Could you check a few things on this model? Use its own coordinates, in mm. Face numbers are marked on the shaded views. A direction names the side the tool comes from. Coordinates: 2 decimals unless noted, no trailing zeros. Write each loop counter-clockwise with the first axis right and the second up, starting at its lowest first coordinate (ties: lowest second). Pieces come first, ordered by that corner, then holes.
Item 1: I want a section at B-B on x = -133.5. Please give me the cut outline in (y, z).
Item 2: Thinking about a two-plate mould opening in Y: for the marked faces 1, 2 and 3, which applies, +Y half, -Y half, draft (parallel to the pull), parting line (faces both ways), or undercut?
Item 3: If I drill on probe 1 along Z at (x, y) = (35, 50); probe 2 along Y at (x, z) = (43.25, 45); probe 3 along X at (y, z) = (156, -101.5), over which ranges is the centre line in solid material (lowest first)?
Item 4: Which directions (+Z, -Z, +X, -X, +Y, -Y) give clear straight access to the entire face, cutting with the end or side of a thin tool? Please do the marked faces 4, 5 and 6.
Item 5: I want a section at C-C on y = -47.5. Please give me the cut outline in (x, z).
Item 6: I want a section at A-A on z = -21. Please give me the cut outline in (x, y), then the cut area to 3 significant figures.
Item 7: I want a section at D-D on z = 52. Please give me the cut outline in (x, y), then the cut area to 3 significant figures.
Item 8: For P1, Ø10, axis at x = -228.5, y = 58, coming from the -Z side; P2, Ø6, axis at y = 89.5, z = -20.5, coming from the +X side; P3, Ø18, axis at x = 1.5, y = 33, coming from the -Z side, each with a flat end and sliding along its axis, tell me the tip position at first contact or that it passes through.
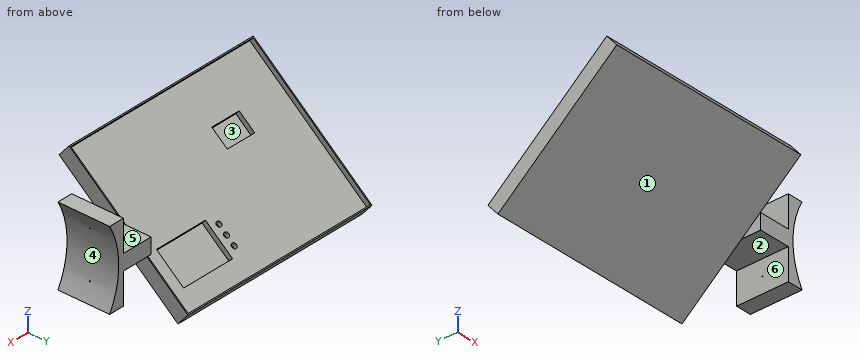
from build123d import *

# Parameters (mm, degrees)
BOSS_EXTRU_1_DEPTH      = 100
BOSS_EXTRU_2_DEPTH      = 400
ESQUISSE3_W             = 396
ESQUISSE3_H             = 296
ESQUISSE3_R             = 5
ESQUISSE3_W_2           = 106.4
ESQUISSE3_H_2           = 68.4
ESQUISSE3_W_3           = 59.5
ESQUISSE3_H_3           = 39
ENL_V_MAT_EXTRU_1_DEPTH = 10
ESQUISSE3_3_W           = 106.4
ESQUISSE3_3_H           = 68.4
ESQUISSE3_3_W_2         = 59.5
ESQUISSE3_3_H_2         = 39
ESQUISSE3_3_R           = 5
ENL_V_MAT_EXTRU_2_DEPTH = 20
ESQUISSE4_R             = 1
ENL_V_MAT_EXTRU_3_DEPTH = 60


with BuildPart() as part:
    # Esquisse1 → Boss.-Extru.1 (new body)
    with BuildSketch(Plane(origin=(0, 0, 0), x_dir=(1, 0, 0), z_dir=(0, 1, 0))):
        with BuildLine():
            Line((30, 15), (30, 75))
            Line((30, 75), (60, 75))
            ThreePointArc((60, 75), (40.208169188, 0), (60, -75))
            Line((60, -75), (30, -75))
            Line((30, -75), (30, -15))
            Line((30, -15), (-30, -15))
            Line((-30, -15), (-30, 15))
            Line((-30, 15), (30, 15))
        make_face()
    extrude(amount=BOSS_EXTRU_1_DEPTH)

    # Esquisse2 → Boss.-Extru.2 (add)
    with BuildSketch(Plane.ZY.offset(30)):
        Polygon((-111.739030315, 152.050914274), (81.097252591, -77.762418662), (104.078585884, -58.478790371), (-88.757697022, 171.334542565), align=None)
    extrude(amount=BOSS_EXTRU_2_DEPTH)

    # Esquisse3 → Enl_v. mat.-Extru.1 (cut)
    with BuildSketch(Plane(origin=(0, 27.086671655, 32.280638256), x_dir=(1, 0, 0), z_dir=(0, 0.64278761, 0.766044443))):
        with Locations((-230, 38.302222156)):
            Rectangle(ESQUISSE3_W, ESQUISSE3_H)
        with Locations((-183.579130296, 134.904442653)):
            Circle(ESQUISSE3_R, mode=Mode.SUBTRACT)
        with Locations((-183.579130296, 115.704442653)):
            Circle(ESQUISSE3_R, mode=Mode.SUBTRACT)
        with Locations((-183.579130296, 96.504442653)):
            Circle(ESQUISSE3_R, mode=Mode.SUBTRACT)
        with Locations((-113.975273558, 115.704442653)):
            Rectangle(ESQUISSE3_W_2, ESQUISSE3_H_2, mode=Mode.SUBTRACT)
        with Locations((-306.627943765, -10.369216509)):
            Rectangle(ESQUISSE3_W_3, ESQUISSE3_H_3, mode=Mode.SUBTRACT)
    extrude(amount=-ENL_V_MAT_EXTRU_1_DEPTH, mode=Mode.SUBTRACT)

    # Esquisse3_3 → Enl_v. mat.-Extru.2 (cut)
    with BuildSketch(Plane(origin=(0, 27.086671655, 32.280638256), x_dir=(1, 0, 0), z_dir=(0, 0.64278761, 0.766044443))):
        with Locations((-113.975273558, 115.704442653)):
            Rectangle(ESQUISSE3_3_W, ESQUISSE3_3_H)
        with Locations((-306.627943765, -10.369216509)):
            Rectangle(ESQUISSE3_3_W_2, ESQUISSE3_3_H_2)
        with Locations((-183.579130296, 96.504442653)):
            Circle(ESQUISSE3_3_R)
        with Locations((-183.579130296, 115.704442653)):
            Circle(ESQUISSE3_3_R)
        with Locations((-183.579130296, 134.904442653)):
            Circle(ESQUISSE3_3_R)
    extrude(amount=-ENL_V_MAT_EXTRU_2_DEPTH, mode=Mode.SUBTRACT)

    # Esquisse4 → Enl_v. mat.-Extru.3 (cut)
    with BuildSketch(Plane.ZY.offset(-30)):
        with Locations((-45, 50)):
            Circle(ESQUISSE4_R)
        with Locations((45, 50)):
            Circle(ESQUISSE4_R)
    extrude(amount=-ENL_V_MAT_EXTRU_3_DEPTH, mode=Mode.SUBTRACT)


solid = part.part
Response values:
1. outline: (-77.76, 81.1) - (152.05, -111.74) - (171.33, -88.76) - (169.8, -87.47) - (163.37, -95.13) - (135.49, -71.74) - (129.06, -79.4) - (76.67, -35.43) - (83.09, -27.77) - (-63.37, 95.13) - (-56.95, 102.79) - (-58.48, 104.08) - close
2. face 1: -Y half
2. face 2: draft
2. face 3: undercut
3. probe 1: z = -75 to -46, -44 to 44, 46 to 75
3. probe 2: y = 0 to 49, 51 to 100
3. probe 3: x = -430 to -30
4. face 4: +X, +Y, -Y
4. face 5: +Z, +Y, -Y
4. face 6: -Z, +Y, -Y
5. outline: (-430, 55.7) - (-30, 55.7) - (-30, 94.87) - (-32, 94.87) - (-32, 81.81) - (-428, 81.81) - (-428, 94.87) - (-430, 94.87) - close
6. outline: (-430, 43.91) - (-30, 43.91) - (-30, 90.58) - (-32, 90.58) - (-32, 75.03) - (-428, 75.03) - (-428, 90.58) - (-430, 90.58) - close; (30, 0) - (41.67, 0) - (41.67, 100) - (30, 100) - close
6. area: 13,700 mm2
7. outline: (-430, -43.09) - (-30, -43.09) - (-30, 3.59) - (-32, 3.59) - (-32, -11.97) - (-428, -11.97) - (-428, 3.59) - (-430, 3.59) - close; (30, 0) - (49.38, 0) - (49.38, 100) - (30, 100) - close
7. area: 14,400 mm2
8. P1: stops at z = -37.02
8. P2: stops at x = 42.04
8. P3: stops at z = -15
